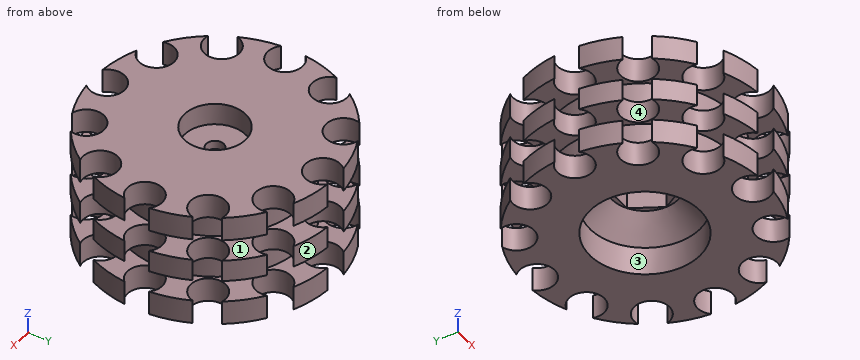
from build123d import *

# Parameters (mm, degrees)
CORTAR_EXTRUIR1_DEPTH   = 9
CROQUIS5_R              = 4
CORTAR_EXTRUIR3_DEPTH   = 27
CROQUIS6_R              = 2
CORTAR_EXTRUIR4_DEPTH   = 10
CROQUIS7_R              = 2
SALIENTE_EXTRUIR1_DEPTH = 1.5
CROQUIS8_R              = 7
CROQUIS8_R_2            = 2
CORTAR_EXTRUIR5_DEPTH   = 1.5


with BuildPart() as part:
    # Croquis1 → Revolución1 (revolve)
    with BuildSketch(Plane(origin=(0, 0, 0), x_dir=(1, 0, 0), z_dir=(0, 1, 0))):
        Polygon((0, 1.5), (0, -9.5), (7, -9.5), (7, -13), (12.5, -13), (27.5, -13), (27.5, -7.5), (20, -7.5), (20, -2.5), (27.5, -2.5), (27.5, 2.5), (20, 2.5), (20, 7.5), (27.5, 7.5), (27.5, 13), (12.5, 13), (12.5, 6.5), (7.5, 1.5), align=None)
    revolve(axis=Axis((0, 0, 0), (0, 0, -1)))

    # Croquis2 → Cortar-Extruir1 (cut)
    with BuildSketch(Plane(origin=(0, 0, -1.5), x_dir=(-1, 0, 0), z_dir=(0, 0, -1))):
        Polygon((7.505553499, 0), (3.75277675, 6.5), (-3.75277675, 6.5), (-7.505553499, 0), (-3.75277675, -6.5), (3.75277675, -6.5), align=None)
    extrude(amount=-CORTAR_EXTRUIR1_DEPTH, mode=Mode.SUBTRACT)

    # Croquis5 → Cortar-Extruir3 (cut, through all)
    with BuildSketch(Plane.XY.offset(13)):
        with Locations((0, 24.5)):
            Circle(CROQUIS5_R)
        with Locations((12.25, 21.217622393)):
            Circle(CROQUIS5_R)
        with Locations((21.217622393, 12.25)):
            Circle(CROQUIS5_R)
        with Locations((24.5, 0)):
            Circle(CROQUIS5_R)
        with Locations((21.217622393, -12.25)):
            Circle(CROQUIS5_R)
        with Locations((12.25, -21.217622393)):
            Circle(CROQUIS5_R)
        with Locations((0, -24.5)):
            Circle(CROQUIS5_R)
        with Locations((-12.25, -21.217622393)):
            Circle(CROQUIS5_R)
        with Locations((-21.217622393, -12.25)):
            Circle(CROQUIS5_R)
        with Locations((-24.5, 0)):
            Circle(CROQUIS5_R)
        with Locations((-21.217622393, 12.25)):
            Circle(CROQUIS5_R)
        with Locations((-12.25, 21.217622393)):
            Circle(CROQUIS5_R)
    extrude(amount=-CORTAR_EXTRUIR3_DEPTH, mode=Mode.SUBTRACT)

    # Croquis6 → Cortar-Extruir4 (cut)
    with BuildSketch(Plane(origin=(0, 0, 7.5), x_dir=(-1, 0, 0), z_dir=(0, 0, -1))):
        Circle(CROQUIS6_R)
    extrude(amount=-CORTAR_EXTRUIR4_DEPTH, mode=Mode.SUBTRACT)

    # Croquis7 → Saliente-Extruir1 (add)
    with BuildSketch(Plane(origin=(0, 0, 7.5), x_dir=(-1, 0, 0), z_dir=(0, 0, -1))):
        Polygon((3.75277675, -6.5), (7.505553499, 0), (3.75277675, 6.5), (-3.75277675, 6.5), (-7.505553499, 0), (-3.75277675, -6.5), align=None)
        Circle(CROQUIS7_R, mode=Mode.SUBTRACT)
    extrude(amount=SALIENTE_EXTRUIR1_DEPTH)

    # Croquis8 → Cortar-Extruir5 (cut)
    with BuildSketch(Plane.XY.offset(9.5)):
        Circle(CROQUIS8_R)
        Circle(CROQUIS8_R_2, mode=Mode.SUBTRACT)
    extrude(amount=-CORTAR_EXTRUIR5_DEPTH, mode=Mode.SUBTRACT)


solid = part.part
Input: part model. Units: mm. Frame: model coordinates. Face numbers are marked on the shaded views. Coordinates: 2 decimals unless noted, no trailing zeros. Loops run counter-clockwise (first coordinate to the right, second up) from the corner with the lowest first, then second, coordinate; pieces in that order, holes last. Notation, with made-up numbers: (65, 34) -> (121, 34) arc R28 ccw to (121, 53) -> close; hole circle Ø8 at (-20, 64). An arc over 180 degrees is marked (long way). Write item = value, one per line. Start each with the question number.
Item 1: Mould query, pull axis Y, two halves, no side actions, for the marked faces 1, 2, 3 and 4. Classes: pulls with the +Y half, pulls with the -Y half, needs draft (parallel to the pull), parting line crosses it, or undercut.
Item 2: Cut plane A-A, the plane z = 10.5. Return loops of the section in (x, y).
Item 3: Cut plane C-C, the plane y = -14.5. Return loops of the section in (x, z).
Item 4: Material intervals for line 1 (Z direction, x = -14, y = -17); line 2 (Y direction, x = -9.5, z = -8.75); line 3 (Y direction, x = -10, z = -10), sorted ascending.
Item 5: Cut plane D-D, the plane x = -10. Count the separate pieces of the cut face and the enclosed holes in it, plus the area to 3 significant figures.
Item 6: First-contact query: P1, Ø8, axis at x = 18, z = -3, coming from the +Y side; P2, Ø6.5, axis at x = -1.5, y = -1.5, coming from the -Z side; P3, Ø1.5, axis at x = 18, z = -2, coming from the +Y side. Flat tips, straight axial feed; report the tip coordinate or a pass-through.
Item 7: Cut plane B-B, the plane y = -23.5. Return loops of the section in (x, z), plus the area to 3 significant figures.
Ans:
q1.face_1 = needs draft
q1.face_2 = pulls with the +Y half
q1.face_3 = undercut
q1.face_4 = undercut
q2.outline = (-27.36, -2.8) arc R27.5 ccw to (-25.09, -11.25) arc R4 cw (long way) to (-22.29, -16.1) arc R27.5 ccw to (-16.1, -22.29) arc R4 cw (long way) to (-11.25, -25.09) arc R27.5 ccw to (-2.8, -27.36) arc R4 cw (long way) to (2.8, -27.36) arc R27.5 ccw to (11.25, -25.09) arc R4 cw (long way) to (16.1, -22.29) arc R27.5 ccw to (22.29, -16.1) arc R4 cw (long way) to (25.09, -11.25) arc R27.5 ccw to (27.36, -2.8) arc R4 cw (long way) to (27.36, 2.8) arc R27.5 ccw to (25.09, 11.25) arc R4 cw (long way) to (22.29, 16.1) arc R27.5 ccw to (16.1, 22.29) arc R4 cw (long way) to (11.25, 25.09) arc R27.5 ccw to (2.8, 27.36) arc R4 cw (long way) to (-2.8, 27.36) arc R27.5 ccw to (-11.25, 25.09) arc R4 cw (long way) to (-16.1, 22.29) arc R27.5 ccw to (-22.29, 16.1) arc R4 cw (long way) to (-25.09, 11.25) arc R27.5 ccw to (-27.36, 2.8) arc R4 cw (long way) to start; hole circle Ø14 at (0, 0)
q3.outline = (-17.91, -13) -> (17.91, -13) -> (17.91, -7.5) -> (13.77, -7.5) -> (13.77, -2.5) -> (17.91, -2.5) -> (17.91, 2.5) -> (13.77, 2.5) -> (13.77, 7.5) -> (17.91, 7.5) -> (17.91, 13) -> (-17.91, 13) -> (-17.91, 7.5) -> (-13.77, 7.5) -> (-13.77, 2.5) -> (-17.91, 2.5) -> (-17.91, -2.5) -> (-13.77, -2.5) -> (-13.77, -7.5) -> (-17.91, -7.5) -> close
q4.line_1 = -13 to -7.5, -2.5 to 2.5, 7.5 to 13
q4.line_2 = -25.81 to -24.12, -18.31 to -8.12, 8.12 to 18.31, 24.12 to 25.81
q4.line_3 = -25.62 to -24.52, -17.91 to -7.5, 7.5 to 17.91, 24.52 to 25.62
q5.separate_pieces = 7
q5.enclosed_holes = 0
q5.area = 833 mm²
q6.P1 = 22.29
q6.P2 = 6
q6.P3 = 21.42
q7.outline = (-8.97, -13) -> (-3.87, -13) -> (-3.87, -7.5) -> (-8.97, -7.5) -> close; (-8.97, -2.5) -> (-3.87, -2.5) -> (-3.87, 2.5) -> (-8.97, 2.5) -> close; (-8.97, 7.5) -> (-3.87, 7.5) -> (-3.87, 13) -> (-8.97, 13) -> close; (3.87, -13) -> (8.97, -13) -> (8.97, -7.5) -> (3.87, -7.5) -> close; (3.87, -2.5) -> (8.97, -2.5) -> (8.97, 2.5) -> (3.87, 2.5) -> close; (3.87, 7.5) -> (8.97, 7.5) -> (8.97, 13) -> (3.87, 13) -> close
q7.area = 163 mm²
